The listing builds one solid part. Answer for the finished solid, in the listing's coordinates (mm). Coordinates: 2 decimals unless noted, no trailing zeros. Order: outer loops, then holes, each group sorted by start corner. A loop starts at its lowest first (then second) coordinate and runs counter-clockwise, first axis right, second up. Notation, with made-up numbers: (67, 75.25) - (96, 75.25) arc R26 ccw to (96, 102.25) - close; hole circle Ø1 at (88.5, 52.5). An arc over 180 degrees is marked (long way). Use one line per item in the form item = value. Start each with the question number.
Item 1: Section A-A, the plane y = -8.5 is taken. Count the separate pieces of the cut face and the enclosed holes in it, and give its area (3 significant figures).
Item 2: Each of these flat-tipped pins is pushed along its axis until it touches: pin 1 Ø7 at (x, z) = (240, 0) entering from +Y; pin 2 Ø1 at (y, z) = (-7.5, -186) entering from -X; pin 3 Ø6 at (y, z) = (4, -95) entering from +X; pin 4 Ø1 at (x, y) = (186, 6.5) entering from -Z. Where does it stop, or does it pass through?
Item 3: Consider line 1 along X through (y, z) = (-2.75, 0); line 2 along Z through (x, y) = (72.5, -4.25); line 3 along Z through (x, y) = (50, -6.75). Determine where each line is inside the solid, lowest interval first. Write a range as [from, to].
Item 4: Section B-B, the plane z = -16 is taken. Write down the section's boundary in (x, y).
Item 5: Section C-C, the plane x = -264 is taken. Write down the section's boundary in (y, z).
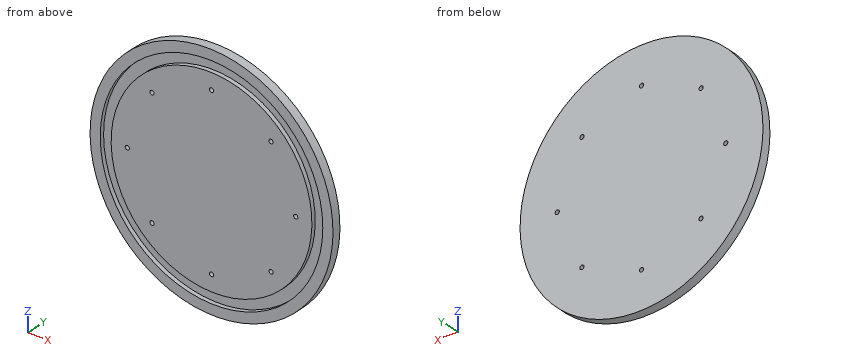
from build123d import *

# Parameters (mm, degrees)
SKETCH1_R           = 346
SKETCH1_R_2         = 6
BOSS_EXTRUDE1_DEPTH = 12.5
SKETCH2_R           = 317
SKETCH2_R_2         = 286
CUT_EXTRUDE1_DEPTH  = 12


with BuildPart() as part:
    # Sketch1 → Boss-Extrude1 (new, symmetric)
    with BuildSketch(Plane(origin=(0, 0, 0), x_dir=(1, 0, 0), z_dir=(0, 1, 0))):
        with Locations(Location((0, 0, 0), (0, 0, 270))):
            Circle(SKETCH1_R)
        with Locations(Location((0, 240, 0), (0, 0, 270))):
            Circle(SKETCH1_R_2, mode=Mode.SUBTRACT)
        with Locations(Location((169.705627485, 169.705627485, 0), (0, 0, 270))):
            Circle(SKETCH1_R_2, mode=Mode.SUBTRACT)
        with Locations(Location((240, 0, 0), (0, 0, 270))):
            Circle(SKETCH1_R_2, mode=Mode.SUBTRACT)
        with Locations(Location((169.705627485, -169.705627485, 0), (0, 0, 270))):
            Circle(SKETCH1_R_2, mode=Mode.SUBTRACT)
        with Locations(Location((0, -240, 0), (0, 0, 270))):
            Circle(SKETCH1_R_2, mode=Mode.SUBTRACT)
        with Locations(Location((-169.705627485, -169.705627485, 0), (0, 0, 270))):
            Circle(SKETCH1_R_2, mode=Mode.SUBTRACT)
        with Locations(Location((-240, 0, 0), (0, 0, 270))):
            Circle(SKETCH1_R_2, mode=Mode.SUBTRACT)
        with Locations(Location((-169.705627485, 169.705627485, 0), (0, 0, 270))):
            Circle(SKETCH1_R_2, mode=Mode.SUBTRACT)
    extrude(amount=BOSS_EXTRUDE1_DEPTH, both=True)

    # Sketch2 → Cut-Extrude1 (cut)
    with BuildSketch(Plane.XZ.offset(12.5)):
        with Locations(Location((0, 0, 0), (0, 0, 270))):
            Circle(SKETCH2_R)
        with Locations(Location((0, 0, 0), (0, 0, 270))):
            Circle(SKETCH2_R_2, mode=Mode.SUBTRACT)
    extrude(amount=-CUT_EXTRUDE1_DEPTH, mode=Mode.SUBTRACT)


solid = part.part
Response:
q1.separate_pieces = 2
q1.enclosed_holes = 9
q1.area = 316,000 mm2
q2.pin_1 = through
q2.pin_2 = -292.07
q2.pin_3 = 333.54
q2.pin_4 = -292.07
q3.line_1 = [-346, -317], [-286, -246], [-234, 234], [246, 286], [317, 346]
q3.line_2 = [-338.32, -308.6], [-276.66, 276.66], [308.6, 338.32]
q3.line_3 = [-342.37, -313.03], [-281.6, 281.6], [313.03, 342.37]
q4.outline = (-345.63, -12.5) - (-316.6, -12.5) - (-316.6, -0.5) - (-285.55, -0.5) - (-285.55, -12.5) - (285.55, -12.5) - (285.55, -0.5) - (316.6, -0.5) - (316.6, -12.5) - (345.63, -12.5) - (345.63, 12.5) - (-345.63, 12.5) - close
q5.outline = (-12.5, -223.65) - (12.5, -223.65) - (12.5, 223.65) - (-12.5, 223.65) - (-12.5, 175.48) - (-0.5, 175.48) - (-0.5, 110) - (-12.5, 110) - (-12.5, -110) - (-0.5, -110) - (-0.5, -175.48) - (-12.5, -175.48) - close
